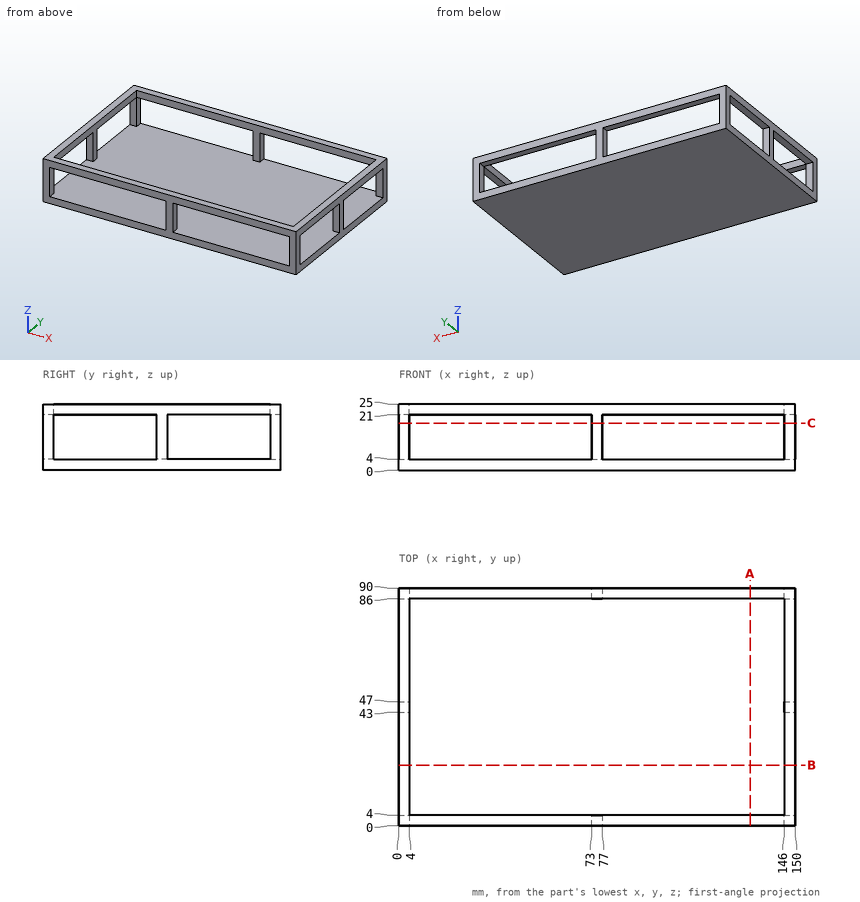
The drawing under review shows one solid part. Ordinate dimensions are in mm from its lowest x, y, z. Round coordinates to 2 decimals unless told otherwise and drop trailing zeros. Write each loop counter-clockwise with the first axis right and the second up, starting at its lowest first coordinate (ties: lowest second). Pieces come first, ordered by that corner, then holes.
(1) Insertion check: pin 1 (5 mm diameter, centred on x = 129.5, y = 55.5, fed in from +Z). The pin has a flat end and moves straight along its axis. Give the tip position at first contact, or say it passes through.
(2) We need section C-C on z = 17.75. Give the number of separate pieces and of enclosed holes in the cut face, and give its area (3 significant figures).
(3) We need section B-B on y = 23. Give the boundary of the cut face in (x, z), and give its area (3 significant figures).
(4) We need section A-A on x = 133. Give the boundary of the cut face in (y, z).
(5) Wall thickness on L1, parallel to X at y = 68, z = 24.25; L2, parallel to Y at x = 97, z = 23; L3, parallel to Z at x = 73.5, y = 26: over which ranges is each line inside the solid? List them lowest first.
Findings below:
1. pin 1: stops at z = 4
2. separate pieces: 8
2. enclosed holes: 0
2. area: 128 mm2
3. outline: (0, 0) - (150, 0) - (150, 4) - (0, 4) - close; (0, 21) - (4, 21) - (4, 25) - (0, 25) - close; (146, 21) - (150, 21) - (150, 25) - (146, 25) - close
3. area: 632 mm2
4. outline: (0, 0) - (90, 0) - (90, 4) - (0, 4) - close; (0, 21) - (4, 21) - (4, 25) - (0, 25) - close; (86, 21) - (90, 21) - (90, 25) - (86, 25) - close
5. L1: x = 0 to 4, 146 to 150
5. L2: y = 0 to 4, 86 to 90
5. L3: z = 0 to 4
